Source: CAD feature listing. Evaluate the final solid. Frame: model axes, mm. A direction names the side the tool comes from. Coordinates: 2 decimals unless noted, no trailing zeros. Loops run counter-clockwise (first coordinate to the right, second up) from the corner with the lowest first, then second, coordinate; pieces in that order, holes last.
from build123d import *

# Parameters (mm, degrees)
PAD_DEPTH       = 2
SKETCH001_R     = 5
PAD001_DEPTH    = 20
SKETCH002_W     = 2
SKETCH002_H     = 15
PAD002_DEPTH    = 15
SKETCH003_R     = 5
SKETCH003_R_2   = 1
PAD003_DEPTH    = 25
SKETCH004_R     = 1
PAD004_DEPTH    = 35
SKETCH005_R     = 3
POCKET_DEPTH    = 2
SKETCH006_R     = 3
POCKET001_DEPTH = 2


with BuildPart() as part:
    # Sketch → Pad (new body)
    with BuildSketch(Plane.XY):
        Polygon((0, 0), (40, 0), (40, 55), (20, 55), (20, 15), (0, 15), align=None)
    extrude(amount=PAD_DEPTH)

    # Sketch001 (on Face8 of Pad) → Pad001 (join)
    with BuildSketch(Plane.XY.offset(2)):
        with Locations((30, 35)):
            Circle(SKETCH001_R)
    extrude(amount=PAD001_DEPTH)

    # Sketch002 (on Face4 of Pad001) → Pad002 (join)
    with BuildSketch(Plane(origin=(0, 0, 0), x_dir=(1, 0, 0), z_dir=(0, 0, -1))):
        with Locations((1, -7.5)):
            Rectangle(SKETCH002_W, SKETCH002_H)
    extrude(amount=PAD002_DEPTH)

    # Sketch003 (on Face10 of Pad002) → Pad003 (join)
    with BuildSketch(Plane(origin=(0, 0, 0), x_dir=(1, 0, 0), z_dir=(0, 0, -1))):
        with Locations((30, -35)):
            Circle(SKETCH003_R)
        with Locations((24, -29)):
            Circle(SKETCH003_R_2)
    extrude(amount=PAD003_DEPTH)

    # Sketch004 (on Face19 of Pad003) → Pad004 (join)
    with BuildSketch(Plane(origin=(0, 0, -25), x_dir=(1, 0, 0), z_dir=(0, 0, -1))):
        with Locations((24, -29)):
            Circle(SKETCH004_R)
        with Locations((30, -35)):
            Circle(SKETCH004_R)
    extrude(amount=PAD004_DEPTH)

    # Sketch005 (on Face1 of Pad004) → Pocket (cut)
    with BuildSketch(Plane.XY.offset(2)):
        with Locations((30, 7.5)):
            Circle(SKETCH005_R)
    extrude(amount=-POCKET_DEPTH, mode=Mode.SUBTRACT)

    # Sketch006 (on Face16 of Pocket) → Pocket001 (cut)
    with BuildSketch(Plane.YZ.offset(2)):
        with Locations((7.5, -7.5)):
            Circle(SKETCH006_R)
    extrude(amount=-POCKET001_DEPTH, mode=Mode.SUBTRACT)


solid = part.part
Q1. Section D-D, the plane x = 34. Return the cut outline in (y, z).
Q2. Line query: line 1 along Z through (x, y) = (0.75, 7.5); line 2 along Y through (x, z) = (30, 1); line 3 along Z through (x, y) = (26, 6.5). Output: solid intervals per line, ascending.
Q3. Section B-B, the plane x = 30. Return the cut outline in (y, z).
Q4. Section C-C, the plane z = -7.5. Return the cut outline in (x, y), plus the area to 3 significant figures.
Q5. Draft query along Y for faces 1 (the cylindrical face through (1.01, 10.36, -6.6)), 2 (the cylindrical face through (27, 7.6, 1)), 3 (the flat face through (5.5, 15, 0.5)), 4 (the flat face through (24, 22, 2)). Return one class per face: +Y half, -Y half, draft (parallel to the pull), parting line (faces both ways), or undercut.
Q6. Section A-A, the plane y = 7.5. Return the cut outline in (x, z), plus the area to 3 significant figures.
Q7. Contact query for flat-ended pins moving along their axis: pin 1 Ø1 at (x, y) = (6, 8) entering from -Z; pin 2 Ø10 at (y, z) = (40.5, -31) entering from -X; pin 3 Ø13.5 at (x, z) = (12, -4) entering from +Y. Output: stop coordinate, or through.
Q8. Access query for faces 5 (the cylindrical face through (30, 34, -42)), 6 (the flat face through (2, 11, -7)), 7 (the cylindrical face through (25, 35, 12)). Directions: +Z, -Z, +X, -X, +Y, -Y. A direction counts if a zero-diameter tool reaches every point of the face in a straight line with its end or side. Return the directions, or none.
Derived:
1. outline: (0, 0) - (32, 0) - (32, -25) - (38, -25) - (38, 0) - (55, 0) - (55, 2) - (38, 2) - (38, 22) - (32, 22) - (32, 2) - (0, 2) - close
2. line 1: z = -15 to -10.5, -4.5 to 2
2. line 2: y = 0 to 4.5, 10.5 to 55
2. line 3: z = 0 to 2
3. outline: (0, 0) - (4.5, 0) - (4.5, 2) - (0, 2) - close; (10.5, 0) - (30, 0) - (30, -25) - (34, -25) - (34, -60) - (36, -60) - (36, -25) - (40, -25) - (40, 0) - (55, 0) - (55, 2) - (40, 2) - (40, 22) - (30, 22) - (30, 2) - (10.5, 2) - close
4. outline: (0, 0) - (2, 0) - (2, 4.5) - (0, 4.5) - close; (0, 10.5) - (2, 10.5) - (2, 15) - (0, 15) - close; circle Ø2 at (24, 29); circle Ø10 at (30, 35)
4. area: 99.7 mm2
5. face 1: undercut
5. face 2: undercut
5. face 3: +Y half
5. face 4: draft
6. outline: (0, -15) - (2, -15) - (2, -10.5) - (0, -10.5) - close; (0, -4.5) - (2, -4.5) - (2, 0) - (27, 0) - (27, 2) - (0, 2) - close; (33, 0) - (40, 0) - (40, 2) - (33, 2) - close
6. area: 86.0 mm2
7. pin 1: stops at z = 0
7. pin 2: stops at x = 29.13
7. pin 3: stops at y = 15
8. face 5: -Z
8. face 6: -Z, +X, +Y, -Y
8. face 7: +Z
